Work out the finished part from the listing and answer in its coordinate system (mm). A direction names the side the tool comes from. Coordinates: 2 decimals unless noted, no trailing zeros. Loops run counter-clockwise (first coordinate to the right, second up) from the corner with the lowest first, then second, coordinate; pieces in that order, holes last. Notation, with made-up numbers: (74.25, -16) - (110.25, -16) arc R22 cw to (110.25, 11) - close; hole circle Ø11 at (-22, -3.5). An arc over 180 degrees is marked (long way). Write each question's results on one line, items separated by ' | '. Start each with the question number.
Item 1: Section B-B, the plane z = 0.55 is taken. Write down the section's boundary in (x, y).
Item 2: Section A-A, the plane y = 20 is taken. Write down the section's boundary in (x, z).
Item 3: A tool of negligible diameter and unlimited length cuts with its end or side. For faces 1 (the face through (26, 0, 2)), 2 (the face through (13, 7, 2)), 3 (the face through (13.5, 6, 2)), from which of +Z, -Z, +X, -X, +Y, -Y can it reach the whole face along a straight path? Write none if from no direction.
Item 4: Consider probe 1 along Y at (x, z) = (25, 1.5); probe 2 along X at (y, z) = (12.5, 0.85); probe 3 along X at (y, z) = (8.25, 0.85). Determine where each line is inside the solid, lowest interval first. Write a range as [from, to].
Item 5: Each of these flat-tipped pins is pushed along its axis until it touches: pin 1 Ø0.9 at (x, z) = (17, 1.5) entering from -Y; pin 2 Ø2.5 at (x, y) = (5, 20) entering from +Z. Where does it stop, or does it pass through?
Item 6: Section C-C, the plane x = 6 is taken. Write down the section's boundary in (y, z).
Item 7: Section D-D, the plane y = 2.5 is taken. Write down the section's boundary in (x, z).
from build123d import *

# Parameters (mm, degrees)
ESQUISSE1_R        = 1.6
BOSS_EXTRU_1_DEPTH = 5


with BuildPart() as part:
    # Esquisse1 → Boss.-Extru.1 (new body)
    with BuildSketch(Plane.XY):
        Polygon((0, 0), (7.5, 0), (7.5, 5), (13.5, 5), (13.5, 7), (12.4, 7), (12.4, 9.3), (13.5, 9.3), (13.5, 13), (16.5, 13), (16.5, 9.3), (17.6, 9.3), (17.6, 7), (16.5, 7), (16.5, 5), (22.5, 5), (22.5, 0), (30, 0), (30, 25), (0, 25), align=None)
        with Locations((5, 10)):
            Circle(ESQUISSE1_R, mode=Mode.SUBTRACT)
        with Locations((5, 20)):
            Circle(ESQUISSE1_R, mode=Mode.SUBTRACT)
        with Locations((25, 10)):
            Circle(ESQUISSE1_R, mode=Mode.SUBTRACT)
        with Locations((15, 20)):
            Circle(ESQUISSE1_R, mode=Mode.SUBTRACT)
        with Locations((25, 20)):
            Circle(ESQUISSE1_R, mode=Mode.SUBTRACT)
    extrude(amount=BOSS_EXTRU_1_DEPTH)


solid = part.part
Answer key:
1) outline: (0, 0) - (7.5, 0) - (7.5, 5) - (13.5, 5) - (13.5, 7) - (12.4, 7) - (12.4, 9.3) - (13.5, 9.3) - (13.5, 13) - (16.5, 13) - (16.5, 9.3) - (17.6, 9.3) - (17.6, 7) - (16.5, 7) - (16.5, 5) - (22.5, 5) - (22.5, 0) - (30, 0) - (30, 25) - (0, 25) - close; hole circle Ø3.2 at (5, 10); hole circle Ø3.2 at (5, 20); hole circle Ø3.2 at (15, 20); hole circle Ø3.2 at (25, 10); hole circle Ø3.2 at (25, 20)
2) outline: (0, 0) - (3.4, 0) - (3.4, 5) - (0, 5) - close; (6.6, 0) - (13.4, 0) - (13.4, 5) - (6.6, 5) - close; (16.6, 0) - (23.4, 0) - (23.4, 5) - (16.6, 5) - close; (26.6, 0) - (30, 0) - (30, 5) - (26.6, 5) - close
3) face 1: +Z, -Z, +X, -X, -Y | face 2: +Z, -Z | face 3: +Z, -Z, -Y
4) probe 1: y = [0, 8.4], [11.6, 18.4], [21.6, 25] | probe 2: x = [0, 13.5], [16.5, 30] | probe 3: x = [0, 12.4], [17.6, 30]
5) pin 1: stops at y = 5 | pin 2: passes through
6) outline: (0, 0) - (8.75, 0) - (8.75, 5) - (0, 5) - close; (11.25, 0) - (18.75, 0) - (18.75, 5) - (11.25, 5) - close; (21.25, 0) - (25, 0) - (25, 5) - (21.25, 5) - close
7) outline: (0, 0) - (7.5, 0) - (7.5, 5) - (0, 5) - close; (22.5, 0) - (30, 0) - (30, 5) - (22.5, 5) - close
